Here's how the part is built. I have some questions about the finished solid (model axes, mm). A direction names the side the tool comes from. Give positions to 0.01 mm unless a question says otherwise; leave off trailing zeros. Loops run counter-clockwise (first coordinate to the right, second up) from the corner with the lowest first, then second, coordinate; pieces in that order, holes last. Notation, with made-up numbers: (88.5, 0) -> (120.5, 0) arc R19 ccw to (120.5, 19) -> close; hole circle Ø4 at (-6.75, 70.5). An arc over 180 degrees is marked (long way). Answer in a Markdown table with one row per item. Add a question column.
Item 1: If we section it at C-C (x = 50): Write out the boundary of the cut face in (y, z) (3 decimals).
Item 2: For P1, Ø1.5, axis at x = 3, y = -9, coming from the -Z side; P2, Ø2, axis at x = 5, z = -11.5, coming from the +Y side; P3, Ø1.5, axis at x = 16, y = -8, coming from the +Z side; P4, Ø7.5, axis at x = 44.45, y = 0, coming from the -Z side, each with a flat end and sliding along its axis, tell me the tip position at first contact or that it passes through.
Item 3: If I drill on line 1 (X direction, y = 0, z = 0.5) (1 decimal); line 2 (Y direction, x = 44.45, z = 2); line 3 (Y direction, x = 44.45, z = 0.5), over which ranges is the centre line in solid material (lowest first)?
Item 4: Which directions (+Z, -Z, +X, -X, +Y, -Y) give clear straight access to the entire face, cutting with the end or side of a thin tool? Please do faces 5 (the face through (6.261, 9.98, -9.356)), 6 (the face through (6.3, -6.9, -11.8)), 7 (the face through (6.261, -6.805, -8.51)), 8 (the face through (6.26, -8.33, 8.45)), 9 (the face through (53.975, 0, 0)).
Item 5: We'd pull the mould along Y, two halves only. Please class faces 1 (the face through (6.261, -10.897, 0.014)), 2 (the face through (6.261, 9.824, 4.715)), 3 (the face through (6.261, 10.897, -0.014)), 4 (the face through (6.261, 4.932, -12.759)): released by +Y, released by -Y, zero draft, split by the parting line, or undercut.
```python
from build123d import *

# Parameters (mm, degrees)
F0_R     = 9.525
F1_DEPTH = 14.3002
F3_DEPTH = 12.7
F4_R     = 9.525
F5_DEPTH = 41.275
F6_R     = 1.1938
F8_R     = 4.7625
F9_DEPTH = 12.7


with BuildPart() as f1:
    # F0 (on Right) → F1 (new body)
    with BuildSketch(Plane.YZ):
        Circle(F0_R)
    extrude(amount=-F1_DEPTH)

    # F2 (on face) → F3 (join)
    with BuildSketch(Plane.YZ):
        with BuildLine():
            Line((1.413542, 12.798762), (0.762, 14.496086))
            ThreePointArc((0.762, 14.496086), (0, 14.5161), (-0.762, 14.496086))
            Line((-0.762, 14.496086), (-1.413542, 12.798762))
            Line((-1.413542, 12.798762), (-1.413542, 10.804526))
            ThreePointArc((-1.413542, 10.804526), (-2.424722, 10.623399), (-3.414351, 10.347855))
            Line((-3.414351, 10.347855), (-4.279618, 12.144599))
            Line((-4.279618, 12.144599), (-5.603078, 13.391142))
            ThreePointArc((-5.603078, 13.391142), (-6.2983, 13.078554), (-6.976154, 12.729903))
            Line((-6.976154, 12.729903), (-6.826732, 10.917973))
            Line((-6.826732, 10.917973), (-5.961465, 9.121229))
            ThreePointArc((-5.961465, 9.121229), (-6.793919, 8.519305), (-7.56599, 7.841663))
            Line((-7.56599, 7.841663), (-9.125146, 9.085049))
            Line((-9.125146, 9.085049), (-10.858397, 9.633918))
            ThreePointArc((-10.858397, 9.633918), (-11.349144, 9.05064), (-11.808596, 8.442406))
            Line((-11.808596, 8.442406), (-10.887804, 6.874746))
            Line((-10.887804, 6.874746), (-9.328648, 5.631361))
            ThreePointArc((-9.328648, 5.631361), (-9.817497, 4.727858), (-10.219092, 3.782335))
            Line((-10.219092, 3.782335), (-12.163328, 4.226094))
            Line((-12.163328, 4.226094), (-13.963078, 3.968578))
            ThreePointArc((-13.963078, 3.968578), (-14.152151, 3.230136), (-14.3022, 2.482788))
            Line((-14.3022, 2.482788), (-12.792413, 1.469891))
            Line((-12.792413, 1.469891), (-10.848177, 1.026132))
            ThreePointArc((-10.848177, 1.026132), (-10.8966, 0), (-10.848177, -1.026132))
            Line((-10.848177, -1.026132), (-12.792413, -1.469891))
            Line((-12.792413, -1.469891), (-14.3022, -2.482788))
            ThreePointArc((-14.3022, -2.482788), (-14.152151, -3.230136), (-13.963078, -3.968578))
            Line((-13.963078, -3.968578), (-12.163328, -4.226094))
            Line((-12.163328, -4.226094), (-10.219092, -3.782335))
            ThreePointArc((-10.219092, -3.782335), (-9.817497, -4.727858), (-9.328648, -5.631361))
            Line((-9.328648, -5.631361), (-10.887804, -6.874746))
            Line((-10.887804, -6.874746), (-11.808596, -8.442406))
            ThreePointArc((-11.808596, -8.442406), (-11.349144, -9.05064), (-10.858397, -9.633918))
            Line((-10.858397, -9.633918), (-9.125146, -9.085049))
            Line((-9.125146, -9.085049), (-7.56599, -7.841663))
            ThreePointArc((-7.56599, -7.841663), (-6.793919, -8.519305), (-5.961465, -9.121229))
            Line((-5.961465, -9.121229), (-6.826732, -10.917973))
            Line((-6.826732, -10.917973), (-6.976154, -12.729903))
            ThreePointArc((-6.976154, -12.729903), (-6.2983, -13.078554), (-5.603078, -13.391142))
            Line((-5.603078, -13.391142), (-4.279618, -12.144599))
            Line((-4.279618, -12.144599), (-3.414351, -10.347855))
            ThreePointArc((-3.414351, -10.347855), (-2.424722, -10.623399), (-1.413542, -10.804526))
            Line((-1.413542, -10.804526), (-1.413542, -12.798762))
            Line((-1.413542, -12.798762), (-0.762, -14.496086))
            ThreePointArc((-0.762, -14.496086), (0, -14.5161), (0.762, -14.496086))
            Line((0.762, -14.496086), (1.413542, -12.798762))
            Line((1.413542, -12.798762), (1.413542, -10.804526))
            ThreePointArc((1.413542, -10.804526), (2.424722, -10.623399), (3.414351, -10.347855))
            Line((3.414351, -10.347855), (4.279618, -12.144599))
            Line((4.279618, -12.144599), (5.603078, -13.391142))
            ThreePointArc((5.603078, -13.391142), (6.2983, -13.078554), (6.976154, -12.729903))
            Line((6.976154, -12.729903), (6.826732, -10.917973))
            Line((6.826732, -10.917973), (5.961465, -9.121229))
            ThreePointArc((5.961465, -9.121229), (6.793919, -8.519305), (7.56599, -7.841663))
            Line((7.56599, -7.841663), (9.125146, -9.085049))
            Line((9.125146, -9.085049), (10.858397, -9.633918))
            ThreePointArc((10.858397, -9.633918), (11.349144, -9.05064), (11.808596, -8.442406))
            Line((11.808596, -8.442406), (10.887804, -6.874746))
            Line((10.887804, -6.874746), (9.328648, -5.631361))
            ThreePointArc((9.328648, -5.631361), (9.817497, -4.727858), (10.219092, -3.782335))
            Line((10.219092, -3.782335), (12.163328, -4.226094))
            Line((12.163328, -4.226094), (13.963078, -3.968578))
            ThreePointArc((13.963078, -3.968578), (14.152151, -3.230136), (14.3022, -2.482788))
            Line((14.3022, -2.482788), (12.792413, -1.469891))
            Line((12.792413, -1.469891), (10.848177, -1.026132))
            ThreePointArc((10.848177, -1.026132), (10.8966, 0), (10.848177, 1.026132))
            Line((10.848177, 1.026132), (12.792413, 1.469891))
            Line((12.792413, 1.469891), (14.3022, 2.482788))
            ThreePointArc((14.3022, 2.482788), (14.152151, 3.230136), (13.963078, 3.968578))
            Line((13.963078, 3.968578), (12.163328, 4.226094))
            Line((12.163328, 4.226094), (10.219092, 3.782335))
            ThreePointArc((10.219092, 3.782335), (9.817497, 4.727858), (9.328648, 5.631361))
            Line((9.328648, 5.631361), (10.887804, 6.874746))
            Line((10.887804, 6.874746), (11.808596, 8.442406))
            ThreePointArc((11.808596, 8.442406), (11.349144, 9.05064), (10.858397, 9.633918))
            Line((10.858397, 9.633918), (9.125146, 9.085049))
            Line((9.125146, 9.085049), (7.56599, 7.841663))
            ThreePointArc((7.56599, 7.841663), (6.793919, 8.519305), (5.961465, 9.121229))
            Line((5.961465, 9.121229), (6.826732, 10.917973))
            Line((6.826732, 10.917973), (6.976154, 12.729903))
            ThreePointArc((6.976154, 12.729903), (6.2983, 13.078554), (5.603078, 13.391142))
            Line((5.603078, 13.391142), (4.279618, 12.144599))
            Line((4.279618, 12.144599), (3.414351, 10.347855))
            ThreePointArc((3.414351, 10.347855), (2.424722, 10.623399), (1.413542, 10.804526))
            Line((1.413542, 10.804526), (1.413542, 12.798762))
        make_face()
    extrude(amount=F3_DEPTH)

    # F4 (on face) → F5 (join)
    with BuildSketch(Plane.YZ.offset(12.7)):
        Circle(F4_R)
    extrude(amount=F5_DEPTH)

    # F6 (on Top) → F7 (revolve, cut)
    with BuildSketch(Plane.XY):
        with Locations((-7.5438, 9.525)):
            Circle(F6_R)
    revolve(axis=Axis((-10.466062, 0, 0), (-1, 0, 0)), mode=Mode.SUBTRACT)

    # F8 (on Top) → F9 (cut, symmetric)
    with BuildSketch(Plane.XY):
        with Locations((44.45, 0)):
            Circle(F8_R)
    extrude(amount=F9_DEPTH, both=True, mode=Mode.SUBTRACT)


solid = f1.part
```
Recorded:
| question | item | result |
|---|---|---|
| 1 | outline | circle Ø19.05 at (0, 0) |
| 2 | P1 | stops at z = -9.28 |
| 2 | P2 | stops at y = 6.96 |
| 2 | P3 | stops at z = 6.18 |
| 2 | P4 | passes through |
| 3 | line 1 | x = -14.3 to 39.7, 49.2 to 54 |
| 3 | line 2 | y = -9.31 to -4.76, 4.76 to 9.31 |
| 3 | line 3 | y = -9.51 to -4.76, 4.76 to 9.51 |
| 4 | face 5 | -Z, +X, -X |
| 4 | face 6 | +X, -X, -Y |
| 4 | face 7 | +X, -X |
| 4 | face 8 | +Z, +X, -X |
| 4 | face 9 | +Z, -Z, +X, +Y, -Y |
| 5 | face 1 | released by -Y |
| 5 | face 2 | undercut |
| 5 | face 3 | released by +Y |
| 5 | face 4 | undercut |
